from build123d import *

# Parameters (mm, degrees)
F0_R      = 69.056327
F1_DEPTH  = 127
F2_R      = 82.153068
F3_DEPTH  = 25.4
F4_R      = 64.976359
F5_DEPTH  = 7.62
F6_W      = 3.676821
F6_H      = 9.284234
F7_DEPTH  = 68.58
F8_W      = 11.629656
F8_H      = 3.530432
F9_DEPTH  = 68.58
F10_W     = 4.776465
F10_H     = 9.760607
F11_DEPTH = 69.85
F12_W     = 4.568793
F12_H     = 9.137589
F13_DEPTH = 69.85


with BuildPart() as f1:
    # F0 (on Top) → F1 (new body)
    with BuildSketch(Plane.XY):
        Circle(F0_R)
    extrude(amount=F1_DEPTH)

    # F2 (on Front) → F3 (cut)
    with BuildSketch(Plane.XZ):
        with Locations((2.311195, 0)):
            Circle(F2_R)
    extrude(amount=-F3_DEPTH, mode=Mode.SUBTRACT)

    # F4 (on face) → F5 (cut)
    with BuildSketch(Plane.XY.offset(127)):
        Circle(F4_R)
    extrude(amount=-F5_DEPTH, mode=Mode.SUBTRACT)

    # F6 (on Front) → F7 (join)
    with BuildSketch(Plane.XZ):
        with Locations((13.182353, 4.642117)):
            Rectangle(F6_W, F6_H)
    extrude(amount=F7_DEPTH)

    # F8 (on Front) → F9 (join)
    with BuildSketch(Plane.XZ):
        with Locations((13.602547, 4.361122)):
            Rectangle(F8_W, F8_H)
    extrude(amount=F9_DEPTH)

    # F10 (on Front) → F11 (join)
    with BuildSketch(Plane.XZ):
        with Locations((8.929915, 15.367763)):
            Rectangle(F10_W, F10_H)
    extrude(amount=F11_DEPTH)

    # F12 (on Front) → F13 (join)
    with BuildSketch(Plane.XZ):
        with Locations((15.886945, 15.679271)):
            Rectangle(F12_W, F12_H)
    extrude(amount=F13_DEPTH)


solid = f1.part
Here's how the part is built. I have some questions about the finished solid (model axes, mm). A direction names the side the tool comes from. Give positions to 0.01 mm unless a question says otherwise; leave off trailing zeros. Loops run counter-clockwise (first coordinate to the right, second up) from the corner with the lowest first, then second, coordinate; pieces in that order, holes last. Notation, with made-up numbers: (82.25, -7) -> (105.25, -7) arc R32 ccw to (105.25, 20) -> close; hole circle Ø8 at (-20.5, -3.75). An arc over 180 degrees is marked (long way). Answer as a JSON object with one key per item and string values. Group by question number.
Item 1: Imagine slicing it at C-C on z = 44.5. Write out the boundary of the cut face in (x, y), then the cut area to 3 significant figures.
Item 2: Imagine slicing it at B-B on x = -40.5. Write out the boundary of the cut face in (y, z).
Item 3: Will these pins go through, and if not, where does the flat tip stop? pin 1 (6 mm diameter, centred on x = 19, y = 16, fed in from +Z); pin 2 (6 mm diameter, centred on x = 51, z = 95, fed in from -Y); pin 3 (1.3 mm diameter, centred on y = -68.5, z = 8, fed in from +X).
Item 4: I need wall thicknesses on L1, parallel to Y at x = 0, z = 125; L2, parallel to Y at x = -1, z = 12.5; L3, parallel to Z at x = 35, y = -54. Which ranges of each line are inside material? Lowest first, please.
Item 5: On a 3-axis mill with a long thin cutter (end or side, diameter ignored), from which of +Z, -Z, +X, -X, +Y, -Y can I reach the whole of each face in a straight line? I mean faces 1 (the cylindrical face through (-14.09, -63.43, 123.24)), 2 (the cylindrical face through (-0.82, 12.522, 82.093)), 3 (the flat face through (16, -69.85, 16)), 4 (the flat face through (14, -68.58, 5)). Say none if no direction works.
Item 6: Thinking about a two-plate mould opening in X: for faces 5 (the flat face through (51, -41, 127)), 6 (the flat face through (-1, 0, 33)), which applies, pulls with the +X half, pulls with the -X half, needs draft (parallel to the pull), parting line crosses it, or undercut?
Item 7: Imagine slicing it at D-D on z = 113.5. Write out the boundary of the cut face in (x, y), then the cut area to 3 significant figures.
Item 8: Imagine slicing it at A-A on y = -55. Write out the boundary of the cut face in (x, z), then the cut area to 3 significant figures.
Answer list:
{
 "1": {"outline": "(-66.75, 0) -> (-66.75, 17.71) arc R69.06 ccw (long way) to (69.06, 0) -> close; (-64.22, 25.4) -> (64.22, 25.4) arc R69.06 ccw to start", "area": "11,600 mm2"},
 "2": {"outline": "(-55.93, 0) -> (0, 0) -> (0, 70.12) -> (25.4, 70.12) -> (25.4, 0) -> (55.93, 0) -> (55.93, 127) -> (50.81, 127) -> (50.81, 119.38) -> (-50.81, 119.38) -> (-50.81, 127) -> (-55.93, 127) -> close"},
 "3": {"pin 1": "stops at z = 119.38", "pin 2": "stops at y = -49.65", "pin 3": "stops at x = 15.02"},
 "4": {"L1": "y = -69.06 to -64.98, 64.98 to 69.06", "L2": "y = -69.05 to 0, 25.4 to 69.05", "L3": "z = 0 to 119.38"},
 "5": {"face 1": "+Z", "face 2": "-Z", "face 3": "+Z, -Z, +X, -X, -Y", "face 4": "-Z, +X, -Y"},
 "6": {"face 5": "needs draft", "face 6": "undercut"},
 "7": {"outline": "circle Ø138.11 at (0, 0)", "area": "15,000 mm2"},
 "8": {"outline": "(-41.76, 0) -> (41.76, 0) -> (41.76, 127) -> (34.6, 127) -> (34.6, 119.38) -> (-34.6, 119.38) -> (-34.6, 127) -> (-41.76, 127) -> close", "area": "10,100 mm2"}
}
